Design review of the part built by this model. Coordinates are the model's own, in mm. Face numbers are marked on the shaded views. A direction names the side the tool comes from. Coordinates: 2 decimals unless noted, no trailing zeros. Order: outer loops, then holes, each group sorted by start corner. A loop starts at its lowest first (then second) coordinate and runs counter-clockwise, first axis right, second up. Notation, with made-up numbers: (8, 82) -> (38, 82) arc R31 ccw to (38, 116) -> close; hole circle Ø10 at (67.5, 43). An arc over 180 degrees is marked (long way). Use a Markdown table: item, result. Add a question column.
Q1. Machinability: for the marked faces 4, 5 and 6, which of the approach directions +Z, -Z, +X, -X, +Y, -Y give a long, thin tool a straight path to every point of the face, cutting with its end or side? Answer none if there is none.
Q2. Insertion check: pin 1 (2 mm diameter, centred on x = -36.5, y = 5, fed in from -Z); pin 2 (3 mm diameter, centred on x = 50.5, y = 3, fed in from -Z); pin 3 (1.5 mm diameter, centred on y = 1.5, z = -43.5, fed in from +X); pin 4 (5.5 mm diameter, centred on x = -32.79, z = 8.49, fed in from -Y). Each pin has a flat end and moves straight along its axis. Give the tip position at first contact, or say it passes through.
Q3. The part is to be moulded in two halves that separate along Z. For the marked faces 1, 2 and 3, say which applies: pulls with the +Z half, pulls with the -Z half, needs draft (parallel to the pull), parting line crosses it, or undercut.
Q4. Add section A-A (z = -10.5). State the section outline as (x, y) points, then the cut area to 3 significant figures.
Q5. Add section B-B (x = -8). Count the separate pieces of the cut face and the enclosed holes in it, then the cut area to 3 significant figures.
Q6. Wall thickness on probe 1 along Z at (x, y) = (47, 3); probe 2 along X at (y, z) = (4, 31); probe 3 along Z at (x, y) = (-4.5, 5.5): over which ranges is each line inside the solid? List them lowest first.
Q7. Add section C-C (x = -56). State the section outline as (y, z) points.
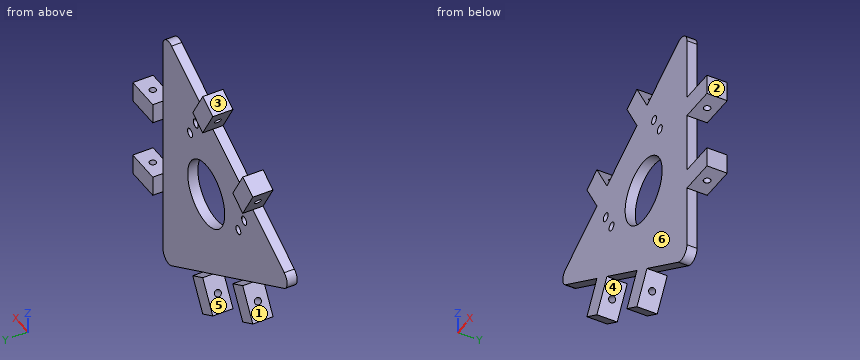
from build123d import *

# Parameters (mm, degrees)
BOSS_EXTRUDE1_DEPTH               = 5
BOSS_EXTRUDE3_DEPTH               = 10
TAP_DRILL_FOR_M4_TAP1_D           = 3.3
TAP_DRILL_FOR_M4_TAP1_CSINK_D     = 3.35
TAP_DRILL_FOR_M4_TAP1_CSINK_ANGLE = 90
CIRPATTERN1_COUNT                 = 3
SKETCH13_R                        = 16
CUT_EXTRUDE1_DEPTH                = 94.577061893
TAP_DRILL_FOR_M5_TAP1_D           = 4.2
TAP_DRILL_FOR_M5_TAP1_CSINK_D     = 4.25
TAP_DRILL_FOR_M5_TAP1_CSINK_ANGLE = 90


with BuildPart() as part:
    # Sketch2 → Boss-Extrude1 (new body)
    with BuildSketch(Plane(origin=(0, 0, 0), x_dir=(0, 0, -1), z_dir=(0, 1, 0))):
        with BuildLine():
            Line((-44.975952642, -2.900635095), (-60.621778265, -30))
            ThreePointArc((-60.621778265, -30), (-60.621778265, -35), (-56.291651246, -37.5))
            Line((-56.291651246, -37.5), (-25, -37.5))
            Line((-25, -37.5), (-15, -37.5))
            Line((-15, -37.5), (15, -37.5))
            Line((15, -37.5), (25, -37.5))
            Line((25, -37.5), (56.291651246, -37.5))
            ThreePointArc((56.291651246, -37.5), (60.621778265, -35), (60.621778265, -30))
            Line((60.621778265, -30), (44.975952642, -2.900635095))
            Line((44.975952642, -2.900635095), (39.975952642, 5.759618943))
            Line((39.975952642, 5.759618943), (24.975952642, 31.740381057))
            Line((24.975952642, 31.740381057), (19.975952642, 40.400635095))
            Line((19.975952642, 40.400635095), (4.330127019, 67.5))
            ThreePointArc((4.330127019, 67.5), (0, 70), (-4.330127019, 67.5))
            Line((-4.330127019, 67.5), (-19.975952642, 40.400635095))
            Line((-19.975952642, 40.400635095), (-24.975952642, 31.740381057))
            Line((-24.975952642, 31.740381057), (-39.975952642, 5.759618943))
            Line((-39.975952642, 5.759618943), (-44.975952642, -2.900635095))
        make_face()
    extrude(amount=BOSS_EXTRUDE1_DEPTH)

    # Sketch2_7 → Boss-Extrude3 (add)
    with BuildSketch(Plane(origin=(0, 0, 0), x_dir=(0, 0, -1), z_dir=(0, 1, 0))):
        Polygon((44.975952642, -2.900635095), (39.975952642, 5.759618943), (54.975952642, 14.419872981), (59.975952642, 5.759618943), align=None)
        Polygon((19.975952642, 40.400635095), (34.975952642, 49.060889132), (39.975952642, 40.400635095), (24.975952642, 31.740381057), align=None)
    boss_extrude3 = extrude(amount=BOSS_EXTRUDE3_DEPTH)

    # Tap Drill for M4 Tap1 (through all)
    with Locations(Plane(origin=(-21.650635095, 0, 12.5), x_dir=(0.49999999999999517, 0, 0.8660254037844415), z_dir=(-0.8660254037844414, 0, 0.4999999999999951))):
        with Locations((-46.160254038, 5)):
            tap_drill_for_m4_tap1 = CounterSinkHole(TAP_DRILL_FOR_M4_TAP1_D / 2, TAP_DRILL_FOR_M4_TAP1_CSINK_D / 2, counter_sink_angle=TAP_DRILL_FOR_M4_TAP1_CSINK_ANGLE)

    # CirPattern1: Boss-Extrude3, Tap Drill for M4 Tap1 ×3 about axis
    cirpattern1_axis = Axis((0, 0, 0), (0, 1, 0))
    add([boss_extrude3.rotate(cirpattern1_axis, i * 360 / CIRPATTERN1_COUNT) for i in range(1, CIRPATTERN1_COUNT)])
    add([tap_drill_for_m4_tap1.rotate(cirpattern1_axis, i * 360 / CIRPATTERN1_COUNT) for i in range(1, CIRPATTERN1_COUNT)], mode=Mode.SUBTRACT)

    # Sketch13 → Cut-Extrude1 (cut, through all)
    with BuildSketch(Plane.XZ):
        with Locations(Location((0.00701443, 0.012149349, 0), (0, 0, 270))):
            Circle(SKETCH13_R)
    extrude(amount=-CUT_EXTRUDE1_DEPTH, mode=Mode.SUBTRACT)

    # Tap Drill for M5 Tap1 (through all)
    with Locations(Plane(origin=(0, 5, 0), x_dir=(1, 0, 0), z_dir=(0, 1, 0))):
        with Locations((-27.789778361, 0.166691947), (-32.789778361, -8.49356209), (14.039248642, -23.983308053), (9.039248642, -32.64356209)):
            CounterSinkHole(TAP_DRILL_FOR_M5_TAP1_D / 2, TAP_DRILL_FOR_M5_TAP1_CSINK_D / 2, counter_sink_angle=TAP_DRILL_FOR_M5_TAP1_CSINK_ANGLE)


solid = part.part
Established:
| question | item | result |
|---|---|---|
| 1 | face 4 | -Z, +Y, -Y |
| 1 | face 5 | -X, +Y, -Y |
| 1 | face 6 | +Z, -Z, +X, -X, -Y |
| 2 | pin 1 | z = -34.95 |
| 2 | pin 2 | z = -25 |
| 2 | pin 3 | x = 37.5 |
| 2 | pin 4 | y = 0 |
| 3 | face 1 | undercut |
| 3 | face 2 | needs draft |
| 3 | face 3 | pulls with the +Z half |
| 4 | outline | (-56.81, 0) -> (-12.06, 0) -> (-12.06, 5) -> (-56.81, 5) -> close; (12.07, 0) -> (37.5, 0) -> (37.5, 5) -> (12.07, 5) -> close |
| 4 | area | 351 mm^2 |
| 5 | separate pieces | 4 |
| 5 | enclosed holes | 2 |
| 5 | area | 525 mm^2 |
| 6 | probe 1 | -25 to -15, 15 to 25 |
| 6 | probe 2 | -46.77 to -41.25, -36 to -35.22, -21.31 to 7.73, 10.35 to 37.5 |
| 6 | probe 3 | -57.79 to -52.52, -48.89 to -40.7, 40.7 to 48.89, 52.52 to 57.79 |
| 7 | outline | (0, -10.97) -> (5, -10.97) -> (5, 10.97) -> (0, 10.97) -> close |
